Autodesk Inventor part; units mm, degrees
ref_plane "YZ Plane" through (0, 0, 0) normal (1, 0, 0) x (0, 1, 0)
ref_plane "XZ Plane" through (0, 0, 0) normal (0, 1, 0) x (-1, 0, 0)
ref_plane "XY Plane" through (0, 0, 0) normal (0, 0, 1) x (1, 0, 0)
sketch "Sketch1" plane through (0, 0, 0) normal (0, 1, 0) x (-1, 0, 0)
  line L0 (2.8823, 56.4) -> (2.8823, -6.592)
  line L1 (-4.4837, -6.592) -> (-4.4837, 56.4)
  line L2 (0.5963, 56.4) -> (0.5963, 51.066)
  line L3 (0.5963, 51.066) -> (-2.1977, 51.066)
  line L4 (-2.1977, 51.066) -> (-2.1977, 56.4)
  line L5 (0.5963, -6.592) -> (0.5963, -1.258)
  line L6 (0.5963, -1.258) -> (-2.1977, -1.258)
  line L7 (-2.1977, -1.258) -> (-2.1977, -6.592)
  line L8 (-4.4837, 56.4) -> (-2.1977, 56.4)
  line L9 (0.5963, 56.4) -> (2.8823, 56.4)
  line L10 (2.8823, -6.592) -> (0.5963, -6.592)
  line L11 (-2.1977, -6.592) -> (-4.4837, -6.592)
  point P0 (0, 0)
  dimension "d0" = 7.366
  dimension "d1" = 62.992
  dimension "d2" = 2.286
  dimension "d3" = 2.286
  dimension "d5" = 2.286
  dimension "d6" = 2.286
  dimension "d7" = 5.334
  dimension "d8" = 5.334
  dimension "d9" = 5.334
  dimension "d10" = 5.334
extrude "Extrusion1" add sketch "Sketch1" along normal blind 66.04
properties part number "ceiling_case_cover"
Read the model definition and answer for the solid it produces. Units are mm, in the model's axes. A direction names the side the tool comes from. Coordinates: 2 decimals unless noted, no trailing zeros. Loops run counter-clockwise (first coordinate to the right, second up) from the corner with the lowest first, then second, coordinate; pieces in that order, holes last.
Q1. Which of the six approach directions +Z, -Z, +X, -X, +Y, -Y give full straight-line access (tool end or side, diameter ignored) to faces 5 (the face through (2.198, 33, -4)), 6 (the face through (1, 0, 25)), 7 (the face through (1, 33, 51.066))?
Q2. The mould has two halves that part along X. Classify faces 1 (the face through (-2, 33, -6.592)), 2 (the face through (-0.596, 33, -4)), 3 (the face through (-0.596, 33, 54)), 4 (the face through (4.484, 33, 24)): +X half, -X half, draft (parallel to the pull), parting line (faces both ways), or undercut.
Q3. The part is cut by section B-B on x = 1. Write down the section's boundary in (y, z).
Q4. This flat-tipped pin is pushed along its axis until it touches: pin 1 Ø0.8 at (x, y) = (0.5, 42.5) entering from +Z. Where does it stop, or does it pass through?
Q5. Consider probe 1 along X at (y, z) = (27, 52); probe 2 along Z at (x, y) = (0, 40). Determine where each line is inside the solid, lowest interval first.
Q6. The part is cut by section A-A on y = 45.5. Write down the section's boundary in (x, z).
Results below:
1. face 5: -Z, +Y, -Y
1. face 6: +Z, -Z, +X, -X, -Y
1. face 7: +Z, +Y, -Y
2. face 1: draft
2. face 2: undercut
2. face 3: undercut
2. face 4: +X half
3. outline: (0, -1.26) - (66.04, -1.26) - (66.04, 51.07) - (0, 51.07) - close
4. pin 1: stops at z = 51.07
5. probe 1: x = -2.88 to -0.6, 2.2 to 4.48
5. probe 2: z = -1.26 to 51.07
6. outline: (-2.88, -6.59) - (-0.6, -6.59) - (-0.6, -1.26) - (2.2, -1.26) - (2.2, -6.59) - (4.48, -6.59) - (4.48, 56.4) - (2.2, 56.4) - (2.2, 51.07) - (-0.6, 51.07) - (-0.6, 56.4) - (-2.88, 56.4) - close
